The model under review builds one solid part; all positions refer to its coordinate system, in mm. A direction names the side the tool comes from. Round coordinates to 2 decimals unless told otherwise and drop trailing zeros. Order: outer loops, then holes, each group sorted by start corner. A loop starts at its lowest first (then second) coordinate and runs counter-clockwise, first axis right, second up. Notation, with made-up numbers: (31, 2.25) -> (36, 2.25) arc R13 cw to (36, 19.25) -> close; hole circle Ø2 at (-34, -26.5). An arc over 180 degrees is marked (long way). Use a Markdown table: item, result. Add a question column.
Autodesk Inventor part; units mm, degrees
ref_plane "YZ Plane" through (0, 0, 0) normal (1, 0, 0) x (0, 1, 0)
ref_plane "XZ Plane" through (0, 0, 0) normal (0, 1, 0) x (-1, 0, 0)
ref_plane "XY Plane" through (0, 0, 0) normal (0, 0, 1) x (1, 0, 0)
sketch "Sketch1" plane through (0, 0, 0) normal (0, 1, 0) x (-1, 0, 0)
  circle A0 centre (0, 0) radius 250
  circle A1 centre (0, 0) radius 200 construction
  line L0 (0, 0) -> (0, -250) construction
  line L1 (0, 0) -> (176.7767, 176.7767) construction
  line L2 (0, 0) -> (250, 0) construction
  line L3 (176.7767, 176.7767) -> (-176.7767, -176.7767) construction
  line L4 (176.7767, -176.7767) -> (-176.7767, 176.7767) construction
  circle A2 centre (141.4214, 141.4214) radius 25
  circle A3 centre (-141.4214, 141.4214) radius 25
  circle A4 centre (-141.4214, -141.4214) radius 25
  circle A5 centre (141.4214, -141.4214) radius 25
  circle A6 centre (200, 0) radius 30
  dimension "d0" = 500
  dimension "d1" = 400
  dimension "d2" = 45
  dimension "d3" = 50
  dimension "d4" = 50
  dimension "d5" = 50
  dimension "d6" = 50
  dimension "d7" = 60
extrude "Extrusion1" add sketch "Sketch1" along normal blind 75
sketch "Sketch2" plane through (0, 75, 0) normal (0, 1, 0) x (1, 0, 0)
  circle A0 centre (0, 0) radius 140
  circle A1 centre (0, 0) radius 92.5
  dimension "d10" = 280
  dimension "d11" = 185
extrude "Extrusion2" add sketch "Sketch2" along normal blind 550
sketch "Sketch4" plane through (0, 625, 0) normal (0, 1, 0) x (1, 0, 0)
  circle A0 centre (0, 0) radius 115
  dimension "d22" = 230
extrude "Extrusion4" cut sketch "Sketch4" against normal blind 100
properties part number "base marcador"
Q1. For pin 1 (2 mm diameter, centred on y = 482.5, z = 129.5, fed in from +X); pin 2 (12 mm diameter, centred on x = 79.5, y = 309, fed in from +Z); pin 3 (10 mm diameter, centred on y = 149.5, z = -18.5, fed in from +X), all flat-tipped, find the tip position at first contact; note any pin that passes through.
Q2. To check wall thickness, follow line 1 along X through (y, z) = (66, -127.5); line 2 along X through (y, z) = (557.5, 0); line 3 along Y through (x, z) = (-33.5, -189). State the ranges of each line that lie inside material, in increasing order.
Q3. Add section B-B, the plane z = 0. Give the boundary of the cut face in (x, y).
Q4. Add section C-C, the plane x = 0. Give the boundary of the cut face in (y, z).
Q5. Add section A-A, the plane x = -200. Give the boundary of the cut face in (y, z).
Q6. For faces 4 (the face through (-121.58, 36.98, 156.63)), 5 (the face through (49.727, 296.85, 77.996)), list the 3-axis set-ups (+Z, -Z, +X, -X, +Y, -Y) from which the entire face can be reached by the end or side of a thin tool; tool diameter is ignored.
Q7. Add section D-D, the plane z = -59.5. Give the boundary of the cut face in (x, y).
Q8. Draft analysis for pull direction X (two halves, no side actions). For faces 1 (the face through (-111.1, 346.15, -85.19)), 2 (the face through (-77, 525, -52)), 3 (the face through (3, 0, 4)), state which applies: released by +X, released by -X, zero draft, split by the parting line, or undercut.
Return value:
| question | item | result |
|---|---|---|
| 1 | pin 1 | x = 55.57 |
| 1 | pin 2 | z = 119.15 |
| 1 | pin 3 | x = 139.35 |
| 2 | line 1 | -215.04 to -162.19, -120.66 to 120.66, 162.19 to 215.04 |
| 2 | line 2 | -140 to -115, 115 to 140 |
| 2 | line 3 | 0 to 75 |
| 3 | outline | (-250, 0) -> (-230, 0) -> (-230, 75) -> (-250, 75) -> close; (-170, 0) -> (250, 0) -> (250, 75) -> (140, 75) -> (140, 625) -> (115, 625) -> (115, 525) -> (92.5, 525) -> (92.5, 75) -> (-92.5, 75) -> (-92.5, 525) -> (-115, 525) -> (-115, 625) -> (-140, 625) -> (-140, 75) -> (-170, 75) -> close |
| 4 | outline | (0, -250) -> (75, -250) -> (75, -140) -> (625, -140) -> (625, -115) -> (525, -115) -> (525, -92.5) -> (75, -92.5) -> (75, 92.5) -> (525, 92.5) -> (525, 115) -> (625, 115) -> (625, 140) -> (75, 140) -> (75, 250) -> (0, 250) -> close |
| 5 | outline | (0, -150) -> (75, -150) -> (75, -30) -> (0, -30) -> close; (0, 30) -> (75, 30) -> (75, 150) -> (0, 150) -> close |
| 6 | face 4 | +Y, -Y |
| 6 | face 5 | +Y |
| 7 | outline | (-242.82, 0) -> (242.82, 0) -> (242.82, 75) -> (126.73, 75) -> (126.73, 625) -> (98.41, 625) -> (98.41, 525) -> (70.82, 525) -> (70.82, 75) -> (-70.82, 75) -> (-70.82, 525) -> (-98.41, 525) -> (-98.41, 625) -> (-126.73, 625) -> (-126.73, 75) -> (-242.82, 75) -> close |
| 8 | face 1 | split by the parting line |
| 8 | face 2 | undercut |
| 8 | face 3 | zero draft |
